Geometry check sheet. Reference: the model listing, model coordinates, mm. Face numbers are marked on the shaded views. Round coordinates to 2 decimals unless told otherwise and drop trailing zeros. Loops run counter-clockwise (first coordinate to the right, second up) from the corner with the lowest first, then second, coordinate; pieces in that order, holes last. Notation, with made-up numbers: (85.5, 12) - (125.5, 12) arc R23 ccw to (125.5, 47) - close; hole circle Ø8 at (10.5, 75.25). An arc over 180 degrees is marked (long way). Answer in a Markdown table with one row per item. Add a question column.
```python
from build123d import *

# Parameters (mm, degrees)
SKETCH1_W           = 11.938
SKETCH1_H           = 11.938
BOSS_EXTRUDE1_DEPTH = 213.106
SKETCH2_R           = 3.68046
BOSS_EXTRUDE2_DEPTH = 22.225
SKETCH3_R           = 3.68046
BOSS_EXTRUDE3_DEPTH = 28.575
SKETCH4_W           = 4.572
SKETCH4_H           = 4.572
BOSS_EXTRUDE4_DEPTH = 15.24


with BuildPart() as part:
    # Sketch1 → Boss-Extrude1 (new body)
    with BuildSketch(Plane(origin=(0, 0, 0), x_dir=(1, 0, 0), z_dir=(0, 1, 0))):
        Rectangle(SKETCH1_W, SKETCH1_H)
    extrude(amount=BOSS_EXTRUDE1_DEPTH)

    # Sketch2 → Boss-Extrude2 (add)
    with BuildSketch(Plane(origin=(0, 213.106, 0), x_dir=(1, 0, 0), z_dir=(0, 1, 0))):
        Circle(SKETCH2_R)
    extrude(amount=BOSS_EXTRUDE2_DEPTH)

    # Sketch3 → Boss-Extrude3 (add)
    with BuildSketch(Plane(origin=(0, 0, 0), x_dir=(-1, 0, 0), z_dir=(0, -1, 0))):
        Circle(SKETCH3_R)
    extrude(amount=BOSS_EXTRUDE3_DEPTH)

    # Sketch4 → Boss-Extrude4 (add)
    with BuildSketch(Plane(origin=(0, 235.331, 0), x_dir=(1, 0, 0), z_dir=(0, 1, 0))):
        Rectangle(SKETCH4_W, SKETCH4_H)
    extrude(amount=BOSS_EXTRUDE4_DEPTH)


solid = part.part
```
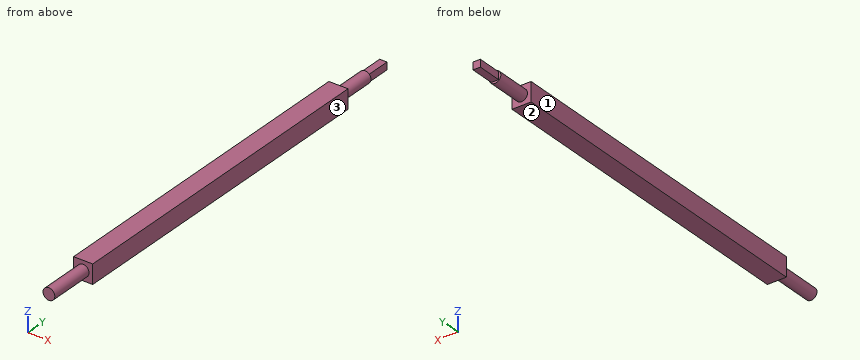
Q1. Depth check by flat-ended pin: P1, Ø2.5, axis at y = 246, z = -1, coming from the +X side; P2, Ø5, axis at x = -2, y = 222.5, coming from the -Z side; P3, Ø3, axis at x = 4, z = 3, coming from the +Y side. Enter the tip coordinate at first touch or a pass-through.
Q2. Cross-section at B-B, the plane z = 0. Enter the section's corners in (x, y) (3 decimals), plus the area to 3 significant figures.
Q3. Cross-section at C-C, the plane y = -9.5. Enter the section's corners in (x, z).
Q4. Scan lines: line 1 (Y direction, x = -4.5, z = 2.25); line 2 (X direction, y = 237, z = 1.75); line 3 (Y direction, x = 2.75, z = -1.5) (3 decimals). Record each from-to range of solid material in increasing order. Write a range as from..to.
Q5. Cross-section at A-A, the plane x = 0. Enter the section's corners in (y, z) (3 decimals).
Q6. Release check for a two-part mould opening along X. For the marked faces 1, 2 and 3 record: +X half, -X half, draft (parallel to the pull), parting line (faces both ways), or undercut.
Check sheet entries:
| question | item | result |
|---|---|---|
| 1 | P1 | x = 2.29 |
| 1 | P2 | z = -3.68 |
| 1 | P3 | y = 235.33 |
| 2 | outline | (-5.969, 0) - (-3.68, 0) - (-3.68, -28.575) - (3.68, -28.575) - (3.68, 0) - (5.969, 0) - (5.969, 213.106) - (3.68, 213.106) - (3.68, 235.331) - (2.286, 235.331) - (2.286, 250.571) - (-2.286, 250.571) - (-2.286, 235.331) - (-3.68, 235.331) - (-3.68, 213.106) - (-5.969, 213.106) - close |
| 2 | area | 2,990 mm² |
| 3 | outline | circle Ø7.36 at (0, 0) |
| 4 | line 1 | 0..213.11 |
| 4 | line 2 | -2.29..2.29 |
| 4 | line 3 | -28.575..235.331 |
| 5 | outline | (-28.575, -3.68) - (0, -3.68) - (0, -5.969) - (213.106, -5.969) - (213.106, -3.68) - (235.331, -3.68) - (235.331, -2.286) - (250.571, -2.286) - (250.571, 2.286) - (235.331, 2.286) - (235.331, 3.68) - (213.106, 3.68) - (213.106, 5.969) - (0, 5.969) - (0, 3.68) - (-28.575, 3.68) - close |
| 6 | face 1 | -X half |
| 6 | face 2 | draft |
| 6 | face 3 | +X half |
